Autodesk Inventor part; units mm, degrees
ref_plane "YZ Plane" through (0, 0, 0) normal (1, 0, 0) x (0, 1, 0)
ref_plane "XZ Plane" through (0, 0, 0) normal (0, 1, 0) x (-1, 0, 0)
ref_plane "XY Plane" through (0, 0, 0) normal (0, 0, 1) x (1, 0, 0)
sketch "Sketch1" plane through (0, 0, 0) normal (0, 1, 0) x (-1, 0, 0)
  line L0 (63.5, 25.4) -> (-63.5, 25.4)
  line L1 (-63.5, 25.4) -> (-63.5, -25.4)
  line L2 (-63.5, -25.4) -> (63.5, -25.4)
  line L3 (63.5, -25.4) -> (63.5, 25.4)
  point P0 (0, 0)
  dimension "d0" = 50.8
  dimension "d1" = 25.4
  dimension "d2" = 63.5
  dimension "d3" = 127
extrude "Extrusion1" add sketch "Sketch1" along normal blind 6.35
sketch "Sketch2" plane through (0, 6.35, 0) normal (0, 1, 0) x (1, 0, 0)
  line L0 (-60.325, -22.225) -> (60.325, -22.225)
  line L1 (60.325, -22.225) -> (60.325, 22.225)
  line L2 (60.325, 22.225) -> (-60.325, 22.225)
  line L3 (-60.325, 22.225) -> (-60.325, -22.225)
  line L4 (-63.5, -25.4) -> (63.5, -25.4)
  line L5 (63.5, -25.4) -> (63.5, 25.4)
  line L6 (63.5, 25.4) -> (-63.5, 25.4)
  line L7 (-63.5, 25.4) -> (-63.5, -25.4)
  point P0 (0, 0)
  dimension "d6" = 3.175
  dimension "d7" = 3.175
  dimension "d8" = 3.175
  dimension "d9" = 3.175
extrude "Extrusion2" add sketch "Sketch2" along normal blind 38.1
fillet "Fillet1" radius 6.35 4 edges at (-60.325, 25.4, -22.225) (60.325, 25.4, -22.225) (60.325, 25.4, 22.225) (-60.325, 25.4, 22.225)
sketch "Sketch4" plane through (63.5, 0, -25.4) normal (0, 0, -1) x (-1, 0, 0)
  line L0 (127, 0) -> (127, 44.45)
  line L1 (127, 44.45) -> (104.775, 44.45)
  line L2 (104.775, 44.45) -> (104.775, 38.1)
  line L3 (104.775, 38.1) -> (127, 38.1)
  line L4 (127, 38.1) -> (127, 44.45)
  line L5 (74.6125, 44.45) -> (52.3875, 44.45)
  line L6 (52.3875, 44.45) -> (52.3875, 38.1)
  line L7 (52.3875, 38.1) -> (74.6125, 38.1)
  line L8 (74.6125, 38.1) -> (74.6125, 44.45)
  line L9 (22.225, 44.45) -> (0, 44.45)
  line L10 (0, 44.45) -> (0, 38.1)
  line L11 (0, 38.1) -> (22.225, 38.1)
  line L12 (22.225, 38.1) -> (22.225, 44.45)
  point P0 (63.5, 0)
  dimension "d28" = 22.225
  dimension "d29" = 6.35
  dimension "d32" = 52.3875
extrude "Extrusion4" [suppressed]
sketch "Sketch5" plane through (-63.5, 0, -25.4) normal (-1, 0, 0) x (0, 0, 1)
  line L0 (-15.24, 38.1) -> (0, 22.86)
  line L1 (0, 0) -> (0, 44.45)
  line L2 (0, 44.45) -> (0, 38.1)
  line L3 (0, 22.86) -> (0, 38.1)
  line L4 (0, 38.1) -> (-15.24, 38.1)
  point P0 (25.4, 0)
  dimension "d39" = 15.24
extrude "Extrusion5" [suppressed]
pattern_linear "Rectangular Pattern1" [suppressed]
pattern_linear "Rectangular Pattern2" [suppressed]
sketch "Sketch6" plane through (-60.325, 38.1, -40.64) normal (0, -1, 0) x (1, 0, 0)
  line L0 (123.825, 15.24) -> (-3.175, 15.24)
  line L1 (15.875, 0) -> (0, 0)
  line L2 (15.875, 0) -> (15.875, 15.24)
  line L3 (0, 15.24) -> (0, 0)
  point P0 (60.325, 40.64)
  point P1 (7.9375, 7.62)
  point P2 (60.3377, 7.62)
  point P3 (112.7379, 7.62)
  dimension "d48" = 7.62
  dimension "d49" = 15.24
  dimension "d50" = 15.875
  dimension "d51" = 7.9375
  dimension "d54" = 52.4002
hole "Hole1" [suppressed]
fillet "Fillet2" [suppressed]
fillet "Fillet3" [suppressed]
mirror "Mirror1" [suppressed]
fillet "Fillet4" [suppressed]
sketch "Sketch13" plane through (0, 44.45, 0) normal (0, 1, 0) x (1, 0, 0)
  line L0 (-74.295, 36.195) -> (74.295, 36.195)
  line L1 (74.295, 36.195) -> (74.295, -36.195)
  line L2 (74.295, -36.195) -> (-74.295, -36.195)
  line L3 (-74.295, -36.195) -> (-74.295, 36.195)
  line L4 (63.5, 25.4) -> (-63.5, 25.4)
  line L5 (-63.5, 25.4) -> (-63.5, -25.4)
  line L6 (-63.5, -25.4) -> (63.5, -25.4)
  line L7 (63.5, -25.4) -> (63.5, 25.4)
  point P0 (0, 0)
  dimension "d81" = 10.795
  dimension "d82" = 10.795
  dimension "d83" = 10.795
  dimension "d84" = 10.795
extrude "Extrusion12" add sketch "Sketch13" against normal blind 6.35
fillet "Fillet6" radius 3.175 4 edges at (-74.295, 41.275, -36.195) (74.295, 41.275, -36.195) (74.295, 41.275, 36.195) (-74.295, 41.275, 36.195)
sketch "Sketch14" plane through (0, 38.1, 0) normal (0, -1, 0) x (1, 0, 0)
  line L0 (74.295, 36.195) -> (-74.295, 36.195)
  line L1 (66.675, 28.575) -> (-66.675, 28.575)
  line L2 (74.295, -36.195) -> (74.295, 36.195)
  line L3 (74.295, -36.195) -> (74.295, 36.195)
  line L4 (74.295, 0) -> (-74.2494, 0) construction
  line L5 (71.12, -36.195) -> (-71.12, -36.195)
  line L6 (66.675, -28.575) -> (66.675, 28.575)
  line L7 (-74.295, -36.195) -> (74.295, -36.195)
  line L8 (0, -36.195) -> (0, 36.195) construction
  point P0 (0, 0)
  point P1 (59.2667, 32.385)
  point P2 (71.12, 36.195)
  point P3 (-71.12, 36.195)
  point P4 (74.295, -33.02)
  point P5 (74.295, 33.02)
  point P6 (44.45, 32.385)
  point P7 (29.6333, 32.385)
  point P8 (14.8167, 32.385)
  point P9 (0, 32.385)
  point P10 (-14.8167, 32.385)
  point P11 (-29.6333, 32.385)
  point P12 (-44.45, 32.385)
  point P13 (-59.2667, 32.385)
  point P14 (59.2667, -32.385)
  point P15 (44.45, -32.385)
  point P16 (29.6333, -32.385)
  point P17 (14.8167, -32.385)
  point P18 (0, -32.385)
  point P19 (-14.8167, -32.385)
  point P20 (-29.6333, -32.385)
  point P21 (-44.45, -32.385)
  point P22 (-59.2667, -32.385)
  point P23 (70.485, -28.956)
  point P24 (70.485, -14.478)
  point P25 (70.485, 0)
  point P26 (70.485, 14.478)
  point P27 (70.485, 28.956)
  point P28 (-70.485, -28.956)
  point P29 (-70.485, -14.478)
  point P30 (-70.485, 0)
  point P31 (-70.485, 14.478)
  point P32 (-70.485, 28.956)
  dimension "d88" = 3.81
  dimension "d89" = 7.62
  dimension "d94" = 14.8167
  dimension "d99" = 118.5333
  dimension "d100" = 59.2667
  dimension "d101" = 7.62
  dimension "d102" = 3.81
  dimension "d103" = 7.239
  dimension "d106" = 14.478
  dimension "d128" = 57.912
  dimension "d129" = 28.956
hole "Hole2" at (59.2667, 38.1, 32.385) at (44.45, 38.1, 32.385) at (29.6333, 38.1, 32.385) at (14.8167, 38.1, 32.385) at (0, 38.1, 32.385) at (-14.8167, 38.1, 32.385) at (-29.6333, 38.1, 32.385) at (-44.45, 38.1, 32.385) at (-59.2667, 38.1, 32.385) at (-59.2667, 38.1, -32.385) at (-44.45, 38.1, -32.385) at (-29.6333, 38.1, -32.385) at (-14.8167, 38.1, -32.385) at (0, 38.1, -32.385) at (14.8167, 38.1, -32.385) at (29.6333, 38.1, -32.385) at (44.45, 38.1, -32.385) at (59.2667, 38.1, -32.385) at (70.485, 38.1, -28.956) at (70.485, 38.1, -14.478) at (70.485, 38.1, 0) at (70.485, 38.1, 14.478) at (70.485, 38.1, 28.956) at (-70.485, 38.1, 28.956) at (-70.485, 38.1, 14.478) at (-70.485, 38.1, 0) at (-70.485, 38.1, -14.478) at (-70.485, 38.1, -28.956) direction (0, 1, 0) diameter 2.9464 depth 25.4 tip angle 118
sketch "Sketch17" plane through (0, 0, 0) normal (0, -1, 0) x (1, 0, 0)
  line L0 (50.4, -14.25) -> (43.6, -14.25)
  line L1 (43.6, -14.25) -> (43.6, 9.75)
  line L2 (43.6, 9.75) -> (50.4, 9.75)
  line L3 (50.4, 9.75) -> (50.4, -14.25)
  point P0 (0, 0)
extrude "Extrusion14" cut sketch "Sketch17" against normal blind 6.35
sketch "Sketch18" plane through (0, 0, 0) normal (0, -1, 0) x (1, 0, 0)
  line L0 (59.29, -7.85) -> (52.49, -7.85)
  line L1 (52.49, -7.85) -> (52.49, 5.95)
  line L2 (52.49, 5.95) -> (59.29, 5.95)
  line L3 (59.29, 5.95) -> (59.29, -7.85)
  line L4 (-56.75, -4.3) -> (-49.95, -4.3)
  line L5 (-49.95, -4.3) -> (-49.95, -14.2)
  line L6 (-49.95, -14.2) -> (-56.75, -14.2)
  line L7 (-56.75, -14.2) -> (-56.75, -4.3)
  point P0 (0, 0)
extrude "Extrusion15" cut sketch "Sketch18" against normal through all
sketch "Sketch19" plane through (0, 0, 0) normal (0, -1, 0) x (1, 0, 0)
  circle A0 centre (55.89, 8.15) radius 1.6
  circle A1 centre (55.89, -10.05) radius 1.6
  circle A2 centre (-53.35, -2.1) radius 1.6
  circle A3 centre (-53.35, -16.4) radius 1.6
  circle A4 centre (47, -16.4) radius 1.6
  circle A5 centre (47, 11.9) radius 1.6
  point P0 (0, 0)
extrude "Extrusion16" cut sketch "Sketch19" against normal through all
sketch "Sketch20" plane through (0, 44.45, 0) normal (0, 1, 0) x (1, 0, 0)
  circle A0 centre (47, 16.4) radius 1.6
  circle A1 centre (-53.35, 2.1) radius 1.6
  circle A2 centre (55.89, -8.15) radius 1.6
  circle A3 centre (55.89, 10.05) radius 1.6
  circle A4 centre (-53.35, 16.4) radius 1.6
  circle A5 centre (47, -11.9) radius 1.6
  line L0 (-56.75, 4.3) -> (-56.75, 14.2)
  line L1 (-56.75, 14.2) -> (-49.95, 14.2)
  line L2 (-49.95, 14.2) -> (-49.95, 4.3)
  line L3 (-49.95, 4.3) -> (-56.75, 4.3)
  line L4 (59.29, 7.85) -> (59.29, -5.95)
  line L5 (59.29, -5.95) -> (52.49, -5.95)
  line L6 (52.49, -5.95) -> (52.49, 7.85)
  line L7 (52.49, 7.85) -> (59.29, 7.85)
  line L8 (50.4, 14.25) -> (50.4, -9.75)
  line L9 (50.4, -9.75) -> (43.6, -9.75)
  line L10 (43.6, -9.75) -> (43.6, 14.25)
  line L11 (43.6, 14.25) -> (50.4, 14.25)
  arc A6 (-60.325, -15.875) -> (-53.975, -22.225) centre (-53.975, -15.875) ccw
  line L12 (-53.975, -22.225) -> (53.975, -22.225)
  arc A7 (53.975, -22.225) -> (60.325, -15.875) centre (53.975, -15.875) ccw
  line L13 (60.325, -15.875) -> (60.325, 15.875)
  arc A8 (60.325, 15.875) -> (53.975, 22.225) centre (53.975, 15.875) ccw
  line L14 (53.975, 22.225) -> (-53.975, 22.225)
  arc A9 (-53.975, 22.225) -> (-60.325, 15.875) centre (-53.975, 15.875) ccw
  line L15 (-60.325, 15.875) -> (-60.325, -15.875)
  line L16 (-53.975, 24.9809) -> (53.975, 24.9809)
  arc A10 (63.0809, 15.875) -> (53.975, 24.9809) centre (53.975, 15.875) ccw
  line L17 (63.0809, 15.875) -> (63.0809, -15.875)
  arc A11 (53.975, -24.9809) -> (63.0809, -15.875) centre (53.975, -15.875) ccw
  line L18 (53.975, -24.9809) -> (-53.975, -24.9809)
  arc A12 (-63.0809, -15.875) -> (-53.975, -24.9809) centre (-53.975, -15.875) ccw
  line L19 (-63.0809, -15.875) -> (-63.0809, 15.875)
  arc A13 (-53.975, 24.9809) -> (-63.0809, 15.875) centre (-53.975, 15.875) ccw
  line L20 (53.975, 28.1559) -> (-53.975, 28.1559)
  arc A14 (-53.975, 28.1559) -> (-66.2559, 15.875) centre (-53.975, 15.875) ccw
  line L21 (-66.2559, 15.875) -> (-66.2559, -15.875)
  arc A15 (-66.2559, -15.875) -> (-53.975, -28.1559) centre (-53.975, -15.875) ccw
  line L22 (-53.975, -28.1559) -> (53.975, -28.1559)
  arc A16 (53.975, -28.1559) -> (66.2559, -15.875) centre (53.975, -15.875) ccw
  line L23 (66.2559, -15.875) -> (66.2559, 15.875)
  arc A17 (66.2559, 15.875) -> (53.975, 28.1559) centre (53.975, 15.875) ccw
  point P0 (0, 0)
  dimension "d130" = 2.7559
  dimension "d131" = 3.175
extrude "Extrusion18" cut sketch "Sketch20" against normal blind 2.032 contours A17 L23 A16 L22 A15 L21 A14 L20
fillet "Fillet7" radius 3.175 4 edges at (-63.5, 19.05, -25.4) (63.5, 19.05, -25.4) (63.5, 19.05, 25.4) (-63.5, 19.05, 25.4)
equation "\"d7\" = d6"
equation "\"d8\" = d6"
equation "\"d9\" = d6"
equation "\"d81\" = d83"
equation "\"d82\" = d83"
equation "\"d84\" = d83"
properties part number "Electronics Box" material "Aluminum 6061"
Build history of the part. All positions in model axes, mm. A direction names the side the tool comes from. Round coordinates to 2 decimals unless told otherwise and drop trailing zeros. Write each loop counter-clockwise with the first axis right and the second up, starting at its lowest first coordinate (ties: lowest second). Pieces come first, ordered by that corner, then holes.
1) 3-axis set-ups, long thin cutter, end or side, ignore diameter. For faces 1 (the cylindrical face through (-58.51, 25.67, 20.32)), 2 (the cylindrical face through (-62.59, 19.32, 24.45)), 3 (the flat face through (56, 3, -7.85)): which of +Z, -Z, +X, -X, +Y, -Y reach the whole face in a straight line?
2) Mould opens along Z. For faces 4 (the cylindrical face through (-62.59, 18.78, -24.45)), 5 (the cylindrical face through (71.79, 41.32, -29.64)), 6 (the cylindrical face through (62.55, 19.32, 24.49)) say: +Z half, -Z half, draft (parallel to the pull), parting line (faces both ways), or undercut.
3) Pin check, flat tips, straight feed: pin 1 (2 mm diameter, centred on x = -11, z = -13.5, fed in from +Y); pin 2 (7 mm diameter, centred on x = 48.5, y = 2.5, fed in from +Z); pin 3 (1.9 mm diameter, centred on x = -53.35, z = -2.1, fed in from +Y); pin 4 (10 mm diameter, centred on y = 24, z = -11.5, fed in from -X). Stop position of each tip, or through.
4) Drill centre lines: probe 1 along Z at (x, y) = (44.45, 41.75) (3 decimals); probe 2 along Z at (x, y) = (-53, 27.5) (3 decimals); probe 3 along X at (y, z) = (25, 14.5) (3 decimals). Where is each one in solid material? Low to high.
5) Band-saw the part on A-A, the plane z = -10.05. Give the number of separate pieces and of enclosed holes in the cut face, and give its area (3 significant figures).
6) Band-saw the part on B-B, the plane x = -44.45. List the corners of the cut face in (y, z) (3 decimals).
7) Band-saw the part on C-C, the plane y = 36. List the corners of the cut face in (x, z) (3 decimals).
Ans:
1. face 1: +Y
1. face 2: +Z, -X, -Y
1. face 3: +Y, -Y
2. face 4: -Z half
2. face 5: undercut
2. face 6: +Z half
3. pin 1: stops at y = 6.35
3. pin 2: stops at z = 25.4
3. pin 3: passes through
3. pin 4: stops at x = -63.5
4. probe 1: z = -36.195 to -33.858, -30.912 to -22.225, 22.225 to 30.912, 33.858 to 36.195
4. probe 2: z = -25.4 to -22.225, 22.225 to 25.4
4. probe 3: x = -63.5 to -60.325, 60.325 to 63.5
5. separate pieces: 4
5. enclosed holes: 0
5. area: 1,070 mm2
6. outline: (0, -25.4) - (38.1, -25.4) - (38.1, -30.912) - (44.45, -30.912) - (44.45, -28.156) - (42.418, -28.156) - (42.418, -24.981) - (44.45, -24.981) - (44.45, -22.225) - (6.35, -22.225) - (6.35, 22.225) - (44.45, 22.225) - (44.45, 24.981) - (42.418, 24.981) - (42.418, 28.156) - (44.45, 28.156) - (44.45, 30.912) - (38.1, 30.912) - (38.1, 25.4) - (0, 25.4) - close; (38.1, -36.195) - (44.45, -36.195) - (44.45, -33.858) - (38.1, -33.858) - close; (38.1, 33.858) - (44.45, 33.858) - (44.45, 36.195) - (38.1, 36.195) - close
7. outline: (-63.5, -22.225) arc R3.175 ccw to (-60.325, -25.4) - (60.325, -25.4) arc R3.175 ccw to (63.5, -22.225) - (63.5, 22.225) arc R3.175 ccw to (60.325, 25.4) - (-60.325, 25.4) arc R3.175 ccw to (-63.5, 22.225) - close; hole (-60.325, -15.875) arc R6.35 ccw to (-53.975, -22.225) - (53.975, -22.225) arc R6.35 ccw to (60.325, -15.875) - (60.325, 15.875) arc R6.35 ccw to (53.975, 22.225) - (-53.975, 22.225) arc R6.35 ccw to (-60.325, 15.875) - close
